Verification items for the finished model (mm, model axes). A direction names the side the tool comes from. Round coordinates to 2 decimals unless told otherwise and drop trailing zeros. Order: outer loops, then holes, each group sorted by start corner. A loop starts at its lowest first (then second) coordinate and runs counter-clockwise, first axis right, second up. Notation, with made-up numbers: (78, -6.5) -> (94, -6.5) arc R25 ccw to (94, 12.5) -> close; hole circle Ø7 at (-3.75, 69.25). An arc over 180 degrees is marked (long way). Write item = value, one per line. Start each with the question number.
from build123d import *

# Parameters (mm, degrees)
BOSS_EXTRUDE1_DEPTH = 5
CUT_EXTRUDE1_DEPTH  = 10


with BuildPart() as part:
    # Sketch1 → Boss-Extrude1 (new body)
    with BuildSketch(Plane.XY):
        Polygon((26, 10), (31, 10), (31, -10), (26, -10), (26, -49.25), (-26, -49.25), (-26, 49.25), (26, 49.25), align=None)
    extrude(amount=BOSS_EXTRUDE1_DEPTH)

    # Sketch2 → Cut-Extrude1 (cut)
    with BuildSketch(Plane(origin=(0, 0, 0), x_dir=(-1, 0, 0), z_dir=(0, 0, -1))):
        Polygon((26, 39.25), (22, 39.25), (22, 40.75), (18.8, 40.75), (18.8, 39.25), (11, 39.25), (11, 35.25), (18.8, 35.25), (18.8, 33.75), (22, 33.75), (22, 35.25), (26, 35.25), align=None)
        Polygon((26, -35.25), (26, -39.25), (22, -39.25), (22, -40.75), (18.8, -40.75), (18.8, -39.25), (11, -39.25), (11, -35.25), (18.8, -35.25), (18.8, -33.75), (22, -33.75), (22, -35.25), align=None)
        Polygon((-26, 35.25), (-26, 39.25), (-22, 39.25), (-22, 40.75), (-18.8, 40.75), (-18.8, 39.25), (-11, 39.25), (-11, 35.25), (-18.8, 35.25), (-18.8, 33.75), (-22, 33.75), (-22, 35.25), align=None)
    extrude(amount=-CUT_EXTRUDE1_DEPTH, mode=Mode.SUBTRACT)


solid = part.part
(1) Cross-section at D-D (y = 37.5). Enter the section's corners in (x, z), and give its area (3 significant figures).
(2) Depth check by flat-ended pin: pin 1 (1.2 mm diameter, centred on y = 37.5, z = 1.5, fed in from +X); pin 2 (1.2 mm diameter, centred on y = -40.5, z = 3, fed in from +X). Enter the tip coordinate at first touch or a pass-through.
(3) Cross-section at C-C (y = 24). Enter the section's corners in (x, z).
(4) Draft check along Y on faces 1 (the flat face through (-24, 35.25, 2)), 2 (the flat face through (-26, 0, 2)), 3 (the flat face through (0, -49.25, 2)). Enter one of: +Y half, -Y half, draft (parallel to the pull), parting line (faces both ways), or undercut.
(5) Cross-section at B-B (x = -12). Enter the section's corners in (y, z), and give its area (4 significant figures).
(6) Scan lines: line 1 along Y through (x, z) = (-20, 3.8); line 2 along Y through (x, z) = (-17.5, 4.85); line 3 along X through (y, z) = (35, 3.25). Record each from-to range of solid material in increasing order. Write a range as from..to.
(7) Set-up check for faces 4 (the flat face through (11, 37, 2)), 5 (the flat face through (-15, -39.25, 2)), 6 (the flat face through (26, -29, 2)), 7 (the flat face through (-20, 40.75, 2)), 8 (the flat face through (26, 44, 2)): record each of +Z, -Z, +X, -X, +Y, -Y from which the full face is reachable in a straight line by a thin tool's end or side.
(8) Cross-section at A-A (x = 20). Enter the section's corners in (y, z), and give its area (4 significant figures).
Outcome:
q1.outline = (-11, 0) -> (11, 0) -> (11, 5) -> (-11, 5) -> close
q1.area = 110 mm^2
q2.pin_1 = 11
q2.pin_2 = 26
q3.outline = (-26, 0) -> (26, 0) -> (26, 5) -> (-26, 5) -> close
q4.face_1 = undercut
q4.face_2 = draft
q4.face_3 = -Y half
q5.outline = (-49.25, 0) -> (-39.25, 0) -> (-39.25, 5) -> (-49.25, 5) -> close; (-35.25, 0) -> (35.25, 0) -> (35.25, 5) -> (-35.25, 5) -> close; (39.25, 0) -> (49.25, 0) -> (49.25, 5) -> (39.25, 5) -> close
q5.area = 452.5 mm^2
q6.line_1 = -49.25..-40.75, -33.75..33.75, 40.75..49.25
q6.line_2 = -49.25..-39.25, -35.25..35.25, 39.25..49.25
q6.line_3 = -26..-22, -18.8..18.8, 22..26
q7.face_4 = +Z, -Z, +X
q7.face_5 = +Z, -Z, -X
q7.face_6 = +Z, -Z, +X, -Y
q7.face_7 = +Z, -Z
q7.face_8 = +Z, -Z, +X, +Y
q8.outline = (-49.25, 0) -> (33.75, 0) -> (33.75, 5) -> (-49.25, 5) -> close; (40.75, 0) -> (49.25, 0) -> (49.25, 5) -> (40.75, 5) -> close
q8.area = 457.5 mm^2
